The listing builds one solid part. Answer for the finished solid, in the listing's coordinates (mm). A direction names the side the tool comes from. Round coordinates to 2 decimals unless told otherwise and drop trailing zeros. Write each loop counter-clockwise with the first axis right and the second up, starting at its lowest first coordinate (ties: lowest second). Pieces come first, ordered by that corner, then holes. Notation, with made-up numbers: (18, 87) - (65, 87) arc R13 ccw to (65, 109) - close; hole circle Ø9 at (-17.5, 31). An arc over 180 degrees is marked (long way). Answer as CSV lines item,"result". Start each with the question number.
Item 1: For a pull along Z with two mould halves and no side action, classify faces 1 (the flat face through (-16, 85, 0)), 2 (the cylindrical face through (-7.75, 83.48, 0.17)), 3 (the flat face through (-16, -11, 12.5)) as pulls with the +Z half, pulls with the -Z half, needs draft (parallel to the pull), parting line crosses it, or undercut.
Item 2: A cutting plane is placed at D-D on y = 29. Determine the outline of the cut face in (x, z), and give its area (3 significant figures).
Item 3: Which of the six approach directions +Z, -Z, +X, -X, +Y, -Y give full straight-line access (tool end or side, diameter ignored) to faces 4 (the flat face through (-16, -11, -12.5)), 5 (the flat face through (-13, 75, 12.5)), 6 (the cylindrical face through (-10, 40, 0)), 7 (the cylindrical face through (-11.497, 40.664, 0.253)), 8 (the flat face through (-8, -3, 0))?
Item 4: A cutting plane is placed at A-A on x = -19.25. Determine the outline of the cut face in (y, z), and give its area (3 significant figures).
Item 5: Flat-ended cylindrical pins translate along their axes: pin 1 (3 mm diameter, centred on x = -4, z = 3.5, fed in from +Y); pin 2 (2 mm diameter, centred on y = 7.5, z = -1.5, fed in from +X); pin 3 (5.5 mm diameter, centred on x = -4, z = 5, fed in from -Y); pin 4 (4 mm diameter, centred on y = 52.5, z = -6.5, fed in from -X). Find the tip coordinate at first contact, or state that the pin passes through.
Item 6: A cutting plane is placed at C-C on x = -1.5. Determine the outline of the cut face in (y, z).
Item 7: A cutting plane is placed at B-B on z = 0. Determine the outline of the cut face in (x, y).
Item 8: Straight lines are drawn through the part: line 1 along Y through (x, z) = (-16.5, 10.5); line 2 along Y through (x, z) = (-3, 8.75); line 3 along X through (y, z) = (-40.5, 7). For each, find the intervals that lie inside material, in ascending order. Write a range as [from, to].
Autodesk Inventor part; units mm, degrees
ref_plane "YZ Plane" through (0, 0, 0) normal (1, 0, 0) x (0, 1, 0)
ref_plane "XZ Plane" through (0, 0, 0) normal (0, 1, 0) x (-1, 0, 0)
ref_plane "XY Plane" through (0, 0, 0) normal (0, 0, 1) x (1, 0, 0)
sketch "草圖1" plane through (0, 0, 0) normal (0, 1, 0) x (-1, 0, 0)
  arc A0 (0, -10) -> (0, 10) centre (0, 0) ccw
  arc A1 (0, -11.5) -> (0, 11.5) centre (0, 0) ccw
  line L0 (0, 11.5) -> (0, 10)
  line L1 (0, -10) -> (0, -11.5)
  dimension "d0" = 20
  dimension "d1" = 23
extrude "擠出1" add sketch "草圖1" along normal blind 40
sketch "草圖2" plane through (0, 40, 0) normal (0, 1, 0) x (1, 0, 0)
  line L0 (0, -11.5) -> (0, -10)
  arc A0 (0, 11.5) -> (0, -11.5) centre (0, 0) ccw
  line L1 (0, 10) -> (0, 11.5)
  line L2 (0, -10) -> (0, 10)
extrude "擠出2" add sketch "草圖2" along normal blind 3
sketch "草圖3" plane through (0, 43, 0) normal (0, 1, 0) x (1, 0, 0)
  arc A0 (0, 7.75) -> (0, -7.75) centre (0, 0) ccw
  line L0 (0, -10) -> (0, 10)
  line L1 (0, -7.75) -> (0, 7.75)
  dimension "d7" = 15.5
extrude "擠出3" cut sketch "草圖3" against normal up to next
sketch "草圖5" plane through (0, 0, 0) normal (0, -1, 0) x (1, 0, 0)
  arc A0 (0, 10) -> (0, -10) centre (0, 0) ccw
  line L0 (0, 10) -> (0, 11.5)
  arc A1 (0, 11.5) -> (0, -11.5) centre (0, 0) ccw
  line L1 (0, -11.5) -> (0, -10)
  line L2 (0, 11.5) -> (0, -11.5)
extrude "擠出4" add sketch "草圖5" along normal blind 3
sketch "草圖7" plane through (0, -3, 0) normal (0, -1, 0) x (1, 0, 0)
  arc A0 (0, 7.75) -> (0, -7.75) centre (0, 0) ccw
  line L0 (0, -11.5) -> (0, 11.5)
  line L1 (0, -7.75) -> (0, 7.75)
  dimension "d13" = 15.5
extrude "擠出5" cut sketch "草圖7" against normal up to next
sketch "草圖9" plane through (0, 0, 0) normal (0, 0, 1) x (1, 0, 0)
  line L0 (0, 43) -> (0, -3) construction
  line L1 (0, -3) -> (-11.2, -3) construction
  line L2 (-11.5, -3) -> (0, -3) construction
  line L3 (-11.2, -3) -> (-11.2, -103) construction
  line L4 (-11.2, -3) -> (-11.2, 17) construction
  line L5 (-11.2, 17) -> (-16.2, 17)
  line L6 (-16.2, 17) -> (-16.2, -123)
  line L7 (-16.2, -123) -> (-11.2, -123)
  line L8 (-11.2, -123) -> (-11.2, 17)
  point P0 (0, 0)
  dimension "d18" = 11.2
  dimension "d19" = 100
  dimension "d20" = 20
  dimension "d21" = 5
  dimension "d22" = 140
  dimension "d23" = 5
extrude "擠出6" add sketch "草圖9" along normal mid plane 25
sketch "草圖11" plane through (0, -3, 0) normal (0, -1, 0) x (1, 0, 0)
  line L0 (-16.2, -12.5) -> (-11.2, -12.5)
  line L1 (-16.2, -12.5) -> (0, -12.5)
  line L2 (-11.2, -12.5) -> (-16.2, -12.5)
  line L3 (-16.2, -12.5) -> (-16.2, 12.5)
  line L4 (-16.2, 12.5) -> (-11.2, 12.5)
  line L5 (-11.2, 12.5) -> (0, 12.5)
  line L6 (0, 12.5) -> (0, 11.5)
  arc A0 (-11.2, -2.6096) -> (0, -11.5) centre (0, 0) ccw
  arc A1 (0, 11.5) -> (-11.2, 2.6096) centre (0, 0) ccw
  line L7 (-11.2, -12.5) -> (-11.2, 12.5)
  line L8 (0, -12.5) -> (0, -11.5)
extrude "擠出7" add sketch "草圖11" against normal blind 20 contours L7 A0 L8 L1 | L5 L6 A1 L7
sketch "草圖12" plane through (-11.2, -123, 12.5) normal (1, 0, 0) x (0, 0, -1)
  line L0 (20.25, 120) -> (4.75, 120) construction
  line L1 (25, 120) -> (0, 120)
  line L2 (0, 0) -> (0, 120)
  line L3 (25, 0) -> (0, 0)
  line L4 (25, 120) -> (25, 0)
  line L5 (0, 120) -> (0, 70) construction
  line L6 (0, 70) -> (25, 70)
  point P0 (12.5, 123)
  dimension "d36" = 50
extrude "擠出9" cut sketch "草圖12" against normal up to next contours L4 L3 L2 L6
sketch "草圖16" plane through (0, 43, 0) normal (0, 1, 0) x (1, 0, 0)
  arc A0 (0, 10) -> (0, -10) centre (0, 0) ccw
  arc A1 (0, 11.5) -> (0, -11.5) centre (0, 0) ccw
  line L0 (0, -11.5) -> (0, -7.75)
  line L1 (0, 7.75) -> (0, 11.5)
extrude "擠出11" add sketch "草圖16" along normal blind 39
sketch "草圖17" plane through (0, 82, 0) normal (0, 1, 0) x (1, 0, 0)
  line L0 (0, -10) -> (0, -7.75)
  arc A0 (0, 7.75) -> (0, -7.75) centre (0, 0) ccw
  line L1 (0, 7.75) -> (0, 10)
  arc A1 (0, 11.5) -> (0, -11.5) centre (0, 0) ccw
  line L2 (0, -11.5) -> (0, -10)
  line L3 (0, 10) -> (0, 11.5)
extrude "擠出12" add sketch "草圖17" along normal blind 3
sketch "草圖18" plane through (0, 85, 0) normal (0, 1, 0) x (1, 0, 0)
  arc A0 (0, 11.5) -> (0, -11.5) centre (0, 0) ccw
  line L0 (0, 11.5) -> (0, 12.5)
  line L1 (-16.2, 12.5) -> (0, 12.5)
  line L2 (-16.2, 12.5) -> (-16.2, -12.5)
  line L3 (-16.2, -12.5) -> (0, -12.5)
  line L4 (0, -12.5) -> (0, -11.5)
extrude "擠出13" add sketch "草圖18" against normal blind 20
sketch "草圖19" plane through (0, 43, 0) normal (0, 1, 0) x (1, 0, 0)
  arc A0 (0, 10) -> (0, -10) centre (0, 0) ccw
  line L0 (0, -10) -> (0, -7.75)
  arc A1 (0, 7.75) -> (0, -7.75) centre (0, 0) ccw
  line L1 (0, 7.75) -> (0, 10)
extrude "擠出14" cut sketch "草圖19" against normal blind 3
sketch "Sketch20" plane through (0, 0, 0) normal (0, 0, 1) x (1, 0, 0)
  line L0 (-11.2, -3) -> (0, -3)
  line L1 (0, 85) -> (-16.2, 85)
  point P0 (0, 0)
  dimension "d52" = 88
sketch "Sketch21" plane through (-16.2, 85, -12.5) normal (-1, 0, 0) x (0, 0, 1)
  line L0 (25, 0) -> (20.25, 0)
  line L1 (0, -20) -> (1, -20)
  line L2 (25, 0) -> (0, 0)
  line L3 (0, 0) -> (0, -20)
  line L4 (0, -20) -> (25, -20)
  line L5 (25, -20) -> (25, 0)
  line L6 (25, -68) -> (25, -138)
  line L7 (0, -138) -> (25, -138)
  line L8 (25, -68) -> (0, -68)
  line L9 (0, -68) -> (0, -138)
  line L10 (0, -138) -> (25, -138)
  line L11 (25, -138) -> (25, -68)
  point P0 (12.5, -85)
extrude "Extrusion15" add sketch "Sketch21" along normal blind 9
properties part number "蓋子加平面2"
Geometry says:
1,face 1,"needs draft"
1,face 2,"undercut"
1,face 3,"pulls with the +Z half"
2,outline,"(0, -11.5) - (0, -10) arc R10 cw to (0, 10) - (0, 11.5) arc R11.5 ccw to start"
2,area,"50.7 mm^2"
3,face 4,"-Z, +X, -X, +Y, -Y"
3,face 5,"+Z, +X, -X, +Y, -Y"
3,face 6,"+X"
3,face 7,"-X"
3,face 8,"+Z, -Z, +X, -Y"
4,outline,"(-53, -12.5) - (17, -12.5) - (17, 12.5) - (-53, 12.5) - close; (65, -12.5) - (85, -12.5) - (85, 12.5) - (65, 12.5) - close"
4,area,"2,250 mm^2"
5,pin 1,"passes through"
5,pin 2,"stops at x = -9.68"
5,pin 3,"stops at y = -3"
5,pin 4,"stops at x = -10.58"
6,outline,"(-3, -12.5) - (17, -12.5) - (17, -11.4) - (65, -11.4) - (65, -12.5) - (85, -12.5) - (85, -7.6) - (82, -7.6) - (82, -9.89) - (0, -9.89) - (0, -7.6) - (-3, -7.6) - close; (-3, 7.6) - (0, 7.6) - (0, 9.89) - (82, 9.89) - (82, 7.6) - (85, 7.6) - (85, 12.5) - (65, 12.5) - (65, 11.4) - (17, 11.4) - (17, 12.5) - (-3, 12.5) - close"
7,outline,"(-25.2, -53) - (-11.2, -53) - (-11.2, -3) - (-7.75, -3) - (-7.75, 0) - (-10, 0) - (-10, 82) - (-7.75, 82) - (-7.75, 85) - (-25.2, 85) - (-25.2, 65) - (-11.5, 65) - (-11.5, 17) - (-25.2, 17) - close"
8,line 1,"y = [-53, 17], [65, 85]"
8,line 2,"y = [-3, 0], [82, 85]"
8,line 3,"x = [-25.2, -11.2]"
